Check sheet for the modelled part. Datum: model origin and axes. Units: mm. Face numbers are marked on the shaded views. A direction names the side the tool comes from. Round coordinates to 2 decimals unless told otherwise and drop trailing zeros. Loops run counter-clockwise (first coordinate to the right, second up) from the corner with the lowest first, then second, coordinate; pieces in that order, holes last. Notation, with made-up numbers: (51.25, -3) -> (93.25, -3) arc R29 ccw to (93.25, 31) -> close; hole circle Ø6 at (-29.75, -2.75). An arc over 180 degrees is marked (long way). One line per question, with ' | ' between items.
Autodesk Inventor part; units mm, degrees
ref_plane "YZ Plane" through (0, 0, 0) normal (1, 0, 0) x (0, 1, 0)
ref_plane "XZ Plane" through (0, 0, 0) normal (0, 1, 0) x (-1, 0, 0)
ref_plane "XY Plane" through (0, 0, 0) normal (0, 0, 1) x (1, 0, 0)
sketch "Sketch14" plane through (0, 0, 0) normal (0, 0, 1) x (1, 0, 0)
  line L0 (0, 0) -> (-20, 0)
  line L1 (-20, 0) -> (-20, 20)
  line L2 (-20, 20) -> (0, 20)
  line L3 (0, 20) -> (0, 0)
  line L4 (-5, 5) -> (-10, 5)
  line L5 (-10, 5) -> (-10, 10)
  line L6 (-10, 10) -> (-5, 10)
  line L7 (-5, 10) -> (-5, 5)
  dimension "d71" = 20
  dimension "d72" = 20
  dimension "d73" = 5
  dimension "d74" = 5
extrude "Extrusion9" add sketch "Sketch14" along normal blind 15 contours L0 L1 L2 L3 | L4 L5 L6 L7
fillet "Fillet1" radius 2 12 edges at (-20, 20, 7.5) (-20, 10, 0) (-20, 0, 7.5) (-20, 10, 15) (0, 10, 15) (-10, 20, 15) (0, 20, 7.5) (-10, 20, 0) (-10, 0, 15) (0, 10, 0) (0, 0, 7.5) (-10, 0, 0)
sketch "Sketch19" plane through (0, 0, 0) normal (0, 0, -1) x (-1, 0, 0)
  line L0 (17, 3) -> (12.5, 3)
  line L1 (12.5, 3) -> (12.5, 7.5)
  line L2 (12.5, 7.5) -> (17, 7.5)
  line L3 (17, 7.5) -> (17, 3)
  point P0 (0, 0)
  point P1 (20, 20)
  dimension "d164" = 4.5
  dimension "d165" = 4.5
extrude "Extrusion15" add sketch "Sketch19" along normal blind 5
chamfer "Chamfer12" distance 1 angle 45 4 edges at (-17, 5.25, -5) (-14.75, 7.5, -5) (-12.5, 5.25, -5) (-14.75, 3, -5)
sketch "Sketch24" plane through (0, 0, 15) normal (0, 0, 1) x (1, 0, 0)
  line L0 (-15, 15) -> (-5, 15)
  line L1 (-5, 15) -> (-5, 5)
  line L2 (-5, 5) -> (-15, 5)
  line L3 (-15, 5) -> (-15, 15)
  point P0 (0, 0)
  dimension "d176" = 10
  dimension "d177" = 10
extrude "Extrusion16" cut sketch "Sketch24" against normal blind 10
chamfer "Chamfer13" distance 1 angle 45 4 edges at (-10, 5, 15) (-5, 10, 15) (-10, 15, 15) (-15, 10, 15)
sketch "Sketch28" plane through (-20, 2, 2) normal (-1, 0, 0) x (0, 0, 1)
  point P0 (-2, -2)
  point P1 (8.5, 8)
hole "Hole15" at (-20, 10, 10.5) direction (1, 0, 0) diameter 4 depth 6 counterbore diameter 5 counterbore depth 4.5
sketch "Sketch29" plane through (0, 2, 13) normal (1, 0, 0) x (0, 0, -1)
  circle A0 centre (2.5, 8) radius 2
  point P0 (13, -2)
hole "Hole16" at (0, 10, 10.5) direction (-1, 0, 0) diameter 4 depth 6 counterbore diameter 5 counterbore depth 4.5
sketch "Sketch30" plane through (-18, 20, 2) normal (0, 1, 0) x (1, 0, 0)
  line L0 (18, 2) -> (-2, 2)
  line L1 (-2, 2) -> (-2, -13)
  line L2 (-2, -13) -> (18, -13)
  line L3 (18, -13) -> (18, 2)
  line L4 (-2, -13) -> (8, -13)
  line L5 (8, -13) -> (8, -8.5)
  line L6 (8, -8.5) -> (-2, -8.5)
  line L7 (-2, -8.5) -> (-2, -13)
  dimension "d226" = 20
  dimension "d227" = 15
  dimension "d228" = 10
  dimension "d229" = 4.5
sketch "Sketch31" plane through (-18, 0, 2) normal (0, -1, 0) x (1, 0, 0)
  line L0 (18, -2) -> (-2, -2)
  line L1 (-2, -2) -> (-2, 13)
  line L2 (-2, 13) -> (18, 13)
  line L3 (18, 13) -> (18, -2)
  line L4 (-2, 13) -> (8, 13)
  line L5 (8, 13) -> (8, 8.5)
  line L6 (8, 8.5) -> (-2, 8.5)
  line L7 (-2, 8.5) -> (-2, 13)
  dimension "d230" = 20
  dimension "d231" = 15
  dimension "d232" = 10
  dimension "d233" = 4.5
hole "Hole17" at (-10, 20, 10.5) direction (0, -1, 0) diameter 4 depth 6 counterbore diameter 5 counterbore depth 4.5
hole "Hole18" at (-10, 0, 10.5) direction (0, 1, 0) diameter 4 depth 6 counterbore diameter 5 counterbore depth 4.5
properties part number "Clamp_Adapter_V1"
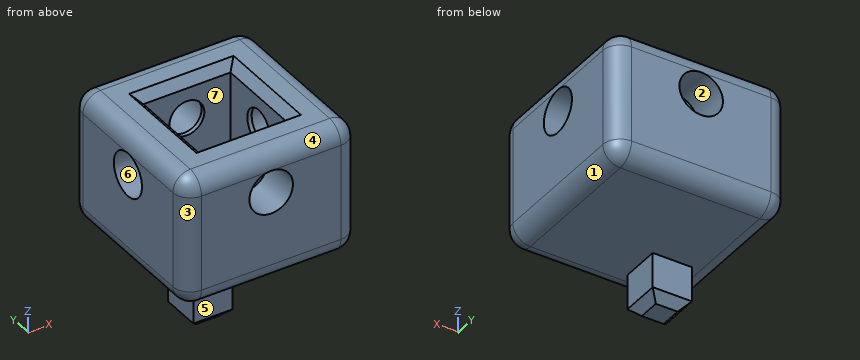
(1) Sectioned sample at D-D, the plane y = 18.5. Record the cut outline in (x, z), and give its area (3 significant figures).
Answer:
outline: (-19.94, 2) arc R1.94 ccw to (-18, 0.06) -> (-2, 0.06) arc R1.94 ccw to (-0.06, 2) -> (-0.06, 13) arc R1.94 ccw to (-2, 14.94) -> (-18, 14.94) arc R1.94 ccw to (-19.94, 13) -> close; hole circle Ø5 at (-10, 10.5) | area: 273 mm2
(2) Sectioned sample at A-A, the plane y = 9.5. Count the separate pieces of the cut face and the enclosed holes in it, and give its area (3 significant figures).
Answer:
separate pieces: 3 | enclosed holes: 0 | area: 148 mm2
(3) Go/stop test with flat-tipped pins: pin 1 (1.5 mm diameter, centred on x = -5.5, y = 6, fed in from -Z); pin 2 (3 mm diameter, centred on y = 4.5, z = -2.5, fed in from -X); pin 3 (2 mm diameter, centred on x = -8.5, y = 8.5, fed in from +Z). Record where each tip stops, or that it passes through.
Answer:
pin 1: stops at z = 0 | pin 2: stops at x = -17 | pin 3: stops at z = 5
(4) Mould release check, pull along Z, two halves, no side actions. Record for the marked faces 1, 2, 3 and 4: +Z half, -Z half, draft (parallel to the pull), parting line (faces both ways), or undercut.
Answer:
face 1: -Z half | face 2: undercut | face 3: draft | face 4: +Z half
(5) Sectioned sample at B-B, the plane x = -6.5. Record the cut outline in (y, z), and give its area (3 significant figures).
Answer:
outline: (0, 2) arc R2 ccw to (2, 0) -> (18, 0) arc R2 ccw to (20, 2) -> (20, 13) arc R2 ccw to (18, 15) -> (16, 15) -> (15, 14) -> (15, 5) -> (5, 5) -> (5, 14) -> (4, 15) -> (2, 15) arc R2 ccw to (0, 13) -> close | area: 196 mm2
(6) Scan lines: probe 1 along Y at (x, z) = (-15.15, 10.5); probe 2 along Y at (x, z) = (-2.25, 10.5); probe 3 along X at (y, z) = (8.5, 5.5). Record each from-to range of solid material in increasing order.
Answer:
probe 1: y = 0 to 8, 12 to 20 | probe 2: y = 0 to 7.5, 12.5 to 20 | probe 3: x = -20 to -15, -5 to 0
(7) Set-up check for the marked faces 5, 6 and 7: record each of +Z, -Z, +X, -X, +Y, -Y from which the full face is reachable in a straight line by a thin tool's end or side.
Answer:
face 5: -Z, +X, -X, -Y | face 6: -X | face 7: +Z
